Source: CAD feature listing. Evaluate the final solid. Frame: model axes, mm. A direction names the side the tool comes from. Coordinates: 2 decimals unless noted, no trailing zeros. Write each loop counter-clockwise with the first axis right and the second up, starting at its lowest first coordinate (ties: lowest second). Pieces come first, ordered by that corner, then holes. Notation, with made-up numbers: (-35, -7) - (24, -7) arc R24 ccw to (24, 11) - close; hole circle Ø6 at (-23.5, 37.25). An arc over 180 degrees is marked (long way). One line per question, with ' | ' between items.
from build123d import *

# Parameters (mm, degrees)
SKETCH030_W     = 37.4
SKETCH030_H     = 41.56
PAD023_DEPTH    = 9
SKETCH031_W     = 28.4
SKETCH031_H     = 27.4
POCKET016_DEPTH = 0.8
SKETCH032_W     = 34.2
SKETCH032_H     = 38.36
POCKET017_DEPTH = 8.2
SKETCH033_W     = 0.9
SKETCH033_H     = 2.6
POCKET018_DEPTH = 8
SKETCH034_W     = 8.5
SKETCH034_H     = 3.4
POCKET019_DEPTH = 5
SKETCH035_W     = 6
SKETCH035_H     = 2.5
PAD024_DEPTH    = 2
SKETCH036_W     = 6
SKETCH036_H     = 2.5
PAD025_DEPTH    = 2
SKETCH037_W     = 20
SKETCH037_H     = 1
PAD026_DEPTH    = 1
SKETCH038_W     = 5
SKETCH038_H     = 1
PAD027_DEPTH    = 1
SKETCH039_W     = 30
SKETCH039_H     = 1
POCKET020_DEPTH = 1
SKETCH040_W     = 30
SKETCH040_H     = 1
POCKET021_DEPTH = 1
SKETCH041_W     = 20
SKETCH041_H     = 1
POCKET022_DEPTH = 1
SKETCH042_W     = 20
SKETCH042_H     = 1
POCKET023_DEPTH = 1


with BuildPart() as part:
    # Sketch030 (on Face1 of ShapeBinder004) → Pad023 (new body)
    with BuildSketch(Plane(origin=(0, 0, -2.3), x_dir=(1, 0, 0), z_dir=(0, 0, -1))):
        with Locations((16.9, -22.98)):
            Rectangle(SKETCH030_W, SKETCH030_H)
    extrude(amount=-PAD023_DEPTH)

    # Sketch031 (on Face5 of Pad023) → Pocket016 (cut)
    with BuildSketch(Plane(origin=(0, 0, -2.3), x_dir=(1, 0, 0), z_dir=(0, 0, -1))):
        with Locations((17, -25.8)):
            Rectangle(SKETCH031_W, SKETCH031_H)
    extrude(amount=-POCKET016_DEPTH, mode=Mode.SUBTRACT)

    # Sketch032 (on Face5 of Pocket016) → Pocket017 (cut)
    with BuildSketch(Plane.XY.offset(6.7)):
        with Locations((16.9, 22.98)):
            Rectangle(SKETCH032_W, SKETCH032_H)
    extrude(amount=-POCKET017_DEPTH, mode=Mode.SUBTRACT)

    # Sketch033 (on Face5 of Pocket017) → Pocket018 (cut)
    with BuildSketch(Plane.XY.offset(6.7)):
        with Locations((34.25, 9.63)):
            Rectangle(SKETCH033_W, SKETCH033_H)
        with Locations((34.25, 36.33)):
            Rectangle(SKETCH033_W, SKETCH033_H)
        with Locations((-0.45, 9.63)):
            Rectangle(SKETCH033_W, SKETCH033_H)
        with Locations((-0.45, 36.33)):
            Rectangle(SKETCH033_W, SKETCH033_H)
    extrude(amount=-POCKET018_DEPTH, mode=Mode.SUBTRACT)

    # Sketch034 (on Face3 of Pocket018) → Pocket019 (cut)
    with BuildSketch(Plane(origin=(35.6, 0, -0.8), x_dir=(0, 1, 0), z_dir=(1, 0, 0))):
        with Locations((22.43, 3.09)):
            Rectangle(SKETCH034_W, SKETCH034_H)
    extrude(amount=-POCKET019_DEPTH, mode=Mode.SUBTRACT)

    # Sketch035 (on Face2 of Pocket019) → Pad024 (join)
    with BuildSketch(Plane(origin=(-1.8, 0, -0.8), x_dir=(0, -1, 0), z_dir=(-1, 0, 0))):
        with Locations((-9.625, 2.8)):
            Rectangle(SKETCH035_W, SKETCH035_H)
        with Locations((-36.335, 2.8)):
            Rectangle(SKETCH035_W, SKETCH035_H)
    extrude(amount=PAD024_DEPTH)

    # Sketch036 (on Face3 of Pad024) → Pad025 (join)
    with BuildSketch(Plane(origin=(35.6, 0, -0.8), x_dir=(0, 1, 0), z_dir=(1, 0, 0))):
        with Locations((9.625, 2.8)):
            Rectangle(SKETCH036_W, SKETCH036_H)
        with Locations((36.335, 2.8)):
            Rectangle(SKETCH036_W, SKETCH036_H)
    extrude(amount=PAD025_DEPTH)

    # Sketch037 (on Face39 of Pad025) → Pad026 (join)
    with BuildSketch(Plane(origin=(0, 42.16, -0.8), x_dir=(1, 0, 0), z_dir=(0, -1, 0))):
        with Locations((16.9, 2.3)):
            Rectangle(SKETCH037_W, SKETCH037_H)
    extrude(amount=PAD026_DEPTH)

    # Sketch038 (on Face31 of Pad026) → Pad027 (join)
    with BuildSketch(Plane(origin=(0, 3.8, -0.8), x_dir=(-1, 0, 0), z_dir=(0, 1, 0))):
        with Locations((-29.3, 2.3)):
            Rectangle(SKETCH038_W, SKETCH038_H)
        with Locations((-4.5, 2.3)):
            Rectangle(SKETCH038_W, SKETCH038_H)
    extrude(amount=PAD027_DEPTH)

    # Sketch039 (on Face39 of Pad027) → Pocket020 (cut)
    with BuildSketch(Plane(origin=(0, 42.16, -0.8), x_dir=(1, 0, 0), z_dir=(0, -1, 0))):
        with Locations((16.9, 6)):
            Rectangle(SKETCH039_W, SKETCH039_H)
    extrude(amount=-POCKET020_DEPTH, mode=Mode.SUBTRACT)

    # Sketch040 (on Face31 of Pocket020) → Pocket021 (cut)
    with BuildSketch(Plane(origin=(0, 3.8, -0.8), x_dir=(-1, 0, 0), z_dir=(0, 1, 0))):
        with Locations((-16.9, 6)):
            Rectangle(SKETCH040_W, SKETCH040_H)
    extrude(amount=-POCKET021_DEPTH, mode=Mode.SUBTRACT)

    # Sketch041 (on Face32 of Pocket021) → Pocket022 (cut)
    with BuildSketch(Plane(origin=(34, 0, -0.8), x_dir=(0, -1, 0), z_dir=(-1, 0, 0))):
        with Locations((-22.98, 6)):
            Rectangle(SKETCH041_W, SKETCH041_H)
    extrude(amount=-POCKET022_DEPTH, mode=Mode.SUBTRACT)

    # Sketch042 (on Face40 of Pocket022) → Pocket023 (cut)
    with BuildSketch(Plane(origin=(-0.2, 0, -0.8), x_dir=(0, 1, 0), z_dir=(1, 0, 0))):
        with Locations((22.98, 6)):
            Rectangle(SKETCH042_W, SKETCH042_H)
    extrude(amount=-POCKET023_DEPTH, mode=Mode.SUBTRACT)


solid = part.part
Item 1: Access query for faces 1 (the face through (31.9, 3, 5)), 2 (the face through (37, 12.625, 2)), 3 (the face through (-3, 36, 3.25)), 4 (the face through (37, 10, 0.75)). Directions: +Z, -Z, +X, -X, +Y, -Y. A direction counts if a zero-diameter tool reaches every point of the face in a straight line with its end or side. Return the directions, or none.
Check sheet entries:
face 1: none | face 2: +Z, -Z, +X | face 3: +Z, -X, +Y, -Y | face 4: -Z, +X, +Y, -Y
Item 2: Ray query, line 1 along Y through (x, z) = (34.5, 2.75); line 2 along X through (y, z) = (14, 5); line 3 along X through (y, z) = (29.5, 4). Return the intervals inside material, ascending. Write a range as [from, to].
Check sheet entries:
line 1: [2.2, 8.33], [10.93, 18.18], [26.68, 35.03], [37.63, 43.76] | line 2: [-1.8, -1.2], [35, 35.6] | line 3: [-1.8, -0.2], [34, 35.6]
Item 3: Cut plane B-B on y = 25. Return loops of the section in (x, z).
Check sheet entries:
outline: (-1.8, -2.3) - (2.8, -2.3) - (2.8, -1.5) - (-0.2, -1.5) - (-0.2, 4.7) - (-1.2, 4.7) - (-1.2, 5.7) - (-0.2, 5.7) - (-0.2, 6.7) - (-1.8, 6.7) - close; (31.2, -2.3) - (35.6, -2.3) - (35.6, 0.59) - (34, 0.59) - (34, -1.5) - (31.2, -1.5) - close; (34, 3.99) - (35.6, 3.99) - (35.6, 6.7) - (34, 6.7) - (34, 5.7) - (35, 5.7) - (35, 4.7) - (34, 4.7) - close
Item 4: Pin query (flat end, axial travel): pin 1 Ø1 at (y, z) = (20, -0.5) entering from +X; pin 2 Ø0.8 at (x, y) = (4.5, 4.5) entering from +Z; pin 3 Ø10 at (x, y) = (10.5, 17) entering from +Z. Return the tip coordinate at first contact, or that it passes through.
Check sheet entries:
pin 1: x = 35.6 | pin 2: z = 2 | pin 3: z = -1.5
Item 5: Cut plane C-C on y = 30.5. Return loops of the section in (x, z).
Check sheet entries:
outline: (-1.8, -2.3) - (2.8, -2.3) - (2.8, -1.5) - (-0.2, -1.5) - (-0.2, 4.7) - (-1.2, 4.7) - (-1.2, 5.7) - (-0.2, 5.7) - (-0.2, 6.7) - (-1.8, 6.7) - close; (31.2, -2.3) - (35.6, -2.3) - (35.6, 6.7) - (34, 6.7) - (34, 5.7) - (35, 5.7) - (35, 4.7) - (34, 4.7) - (34, -1.5) - (31.2, -1.5) - close
Item 6: Cut plane D-D on z = 0. Return loops of the section in (x, y).
Check sheet entries:
outline: (-1.8, 2.2) - (35.6, 2.2) - (35.6, 43.76) - (-1.8, 43.76) - close; hole (-0.9, 8.33) - (-0.2, 8.33) - (-0.2, 3.8) - (34, 3.8) - (34, 8.33) - (34.7, 8.33) - (34.7, 10.93) - (34, 10.93) - (34, 35.03) - (34.7, 35.03) - (34.7, 37.63) - (34, 37.63) - (34, 42.16) - (-0.2, 42.16) - (-0.2, 37.63) - (-0.9, 37.63) - (-0.9, 35.03) - (-0.2, 35.03) - (-0.2, 10.93) - (-0.9, 10.93) - close
Item 7: Cut plane A-A on x = 24. Return loops of the section in (y, z), and give its area (3 significant figures).
Check sheet entries:
outline: (2.2, -2.3) - (12.1, -2.3) - (12.1, -1.5) - (3.8, -1.5) - (3.8, 4.7) - (2.8, 4.7) - (2.8, 5.7) - (3.8, 5.7) - (3.8, 6.7) - (2.2, 6.7) - close; (39.5, -2.3) - (43.76, -2.3) - (43.76, 6.7) - (42.16, 6.7) - (42.16, 5.7) - (43.16, 5.7) - (43.16, 4.7) - (42.16, 4.7) - (42.16, 2) - (41.16, 2) - (41.16, 1) - (42.16, 1) - (42.16, -1.5) - (39.5, -1.5) - close | area: 36.6 mm²
Item 8: Mould query, pull axis Y, two halves, no side actions, for faces 5 (the face through (-3, 39.335, 2)), 6 (the face through (37, 36, 3.25)), 7 (the face through (-1, 23, 5.7)), 8 (the face through (-1.8, 23, 2)). Classes: pulls with the +Y half, pulls with the -Y half, needs draft (parallel to the pull), parting line crosses it, or undercut.
Check sheet entries:
face 5: pulls with the +Y half | face 6: needs draft | face 7: undercut | face 8: undercut
